Geometry check sheet. Reference: the model listing, model coordinates, mm. Face numbers are marked on the shaded views. A direction names the side the tool comes from. Round coordinates to 2 decimals unless told otherwise and drop trailing zeros. Write each loop counter-clockwise with the first axis right and the second up, starting at its lowest first coordinate (ties: lowest second). Pieces come first, ordered by that corner, then holes. Notation, with made-up numbers: (-5.75, 41) -> (47.25, 41) arc R24 ccw to (47.25, 66) -> close; hole circle Ø11 at (-28, 8). An arc over 180 degrees is marked (long way). One line per question, with ' | ' between items.
```python
from build123d import *

# Parameters (mm, degrees)
BOSS_EXTRUDE1_DEPTH       = 5
CUT_EXTRUDE1_DEPTH        = 0.5
CUT_EXTRUDE2_DEPTH        = 3
M3X0_5_TAPPED_HOLE1_D     = 2.5
M3X0_5_TAPPED_HOLE1_DEPTH = 7.5
M3X0_5_TAPPED_HOLE1_TIP   = 0.751075774
FILLET1_R                 = 0.5


with BuildPart() as part:
    # Sketch1 → Boss-Extrude1 (new body)
    with BuildSketch(Plane(origin=(0, 0, 0), x_dir=(1, 0, 0), z_dir=(0, 1, 0))):
        with BuildLine():
            Line((-30, 11), (-6, 11))
            Line((-6, 11), (-6, 0))
            ThreePointArc((-6, 0), (0, -6), (6, 0))
            Line((6, 0), (6, 11))
            Line((6, 11), (40, 11))
            Line((40, 11), (40, -14))
            Line((40, -14), (-30, -14))
            Line((-30, -14), (-30, -2.5))
            Line((-30, -2.5), (-22, -2.5))
            ThreePointArc((-22, -2.5), (-19.5, 0), (-22, 2.5))
            Line((-22, 2.5), (-30, 2.5))
            Line((-30, 2.5), (-30, 11))
        make_face()
        with BuildLine():
            Line((22, 2.5), (30, 2.5))
            ThreePointArc((30, 2.5), (32.5, 0), (30, -2.5))
            Line((30, -2.5), (22, -2.5))
            ThreePointArc((22, -2.5), (19.5, 0), (22, 2.5))
        make_face(mode=Mode.SUBTRACT)
    extrude(amount=BOSS_EXTRUDE1_DEPTH)

    # Sketch2 → Cut-Extrude1 (cut)
    with BuildSketch(Plane.XZ):
        with BuildLine():
            Line((-9, 0), (-9, -11))
            Line((-9, -11), (9, -11))
            Line((9, -11), (9, 0))
            ThreePointArc((9, 0), (0, 9), (-9, 0))
        make_face()
    extrude(amount=-CUT_EXTRUDE1_DEPTH, mode=Mode.SUBTRACT)

    # Sketch3 → Cut-Extrude2 (cut)
    with BuildSketch(Plane.XZ):
        with BuildLine():
            Line((-11, 8), (-11, -5))
            ThreePointArc((-11, -5), (-14, -8), (-17, -5))
            Line((-17, -5), (-17, 8))
            ThreePointArc((-17, 8), (-14, 11), (-11, 8))
        make_face()
        with BuildLine():
            Line((18, 8), (18, -5))
            ThreePointArc((18, -5), (14.5, -8.5), (11, -5))
            Line((11, -5), (11, 8))
            ThreePointArc((11, 8), (14.5, 11.5), (18, 8))
        make_face()
        with BuildLine():
            Line((38.85, 7.5), (38.85, -5))
            ThreePointArc((38.85, -5), (36.35, -7.5), (33.85, -5))
            Line((33.85, -5), (33.85, 7.5))
            ThreePointArc((33.85, 7.5), (36.35, 10), (38.85, 7.5))
        make_face()
    extrude(amount=-CUT_EXTRUDE2_DEPTH, mode=Mode.SUBTRACT)

    # M3x0.5 Tapped Hole1
    with Locations(Plane.XY.offset(14)):
        with Locations((30, 2.5)):
            Hole(M3X0_5_TAPPED_HOLE1_D / 2, depth=M3X0_5_TAPPED_HOLE1_DEPTH)
            with Locations((0, 0, -(M3X0_5_TAPPED_HOLE1_DEPTH + M3X0_5_TAPPED_HOLE1_TIP / 2))):  # 118° drill point
                Cone(0, M3X0_5_TAPPED_HOLE1_D / 2, M3X0_5_TAPPED_HOLE1_TIP, mode=Mode.SUBTRACT)

    # Fillet1
    fillet1_edges = [part.edges().sort_by_distance(p)[0] for p in [
        (40, 2.5, -11),
        (40, 2.5, 14),
        (-30, 2.5, 14),
        (-30, 2.5, -11),
        (-6, 2.75, -11),
        (6, 2.75, -11),
    ]]
    fillet(fillet1_edges, radius=FILLET1_R)


solid = part.part
```
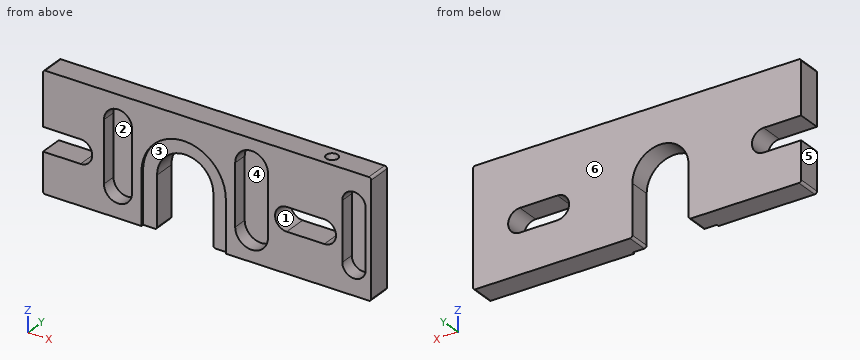
(1) Access from +Z, -Z, +X, -X, +Y, -Y to the whole of each face (thin tool, end or side, straight path). Record for the marked faces 1, 2 and 3.
Resolved:
face 1: +Y, -Y | face 2: -Y | face 3: -Z, -Y
(2) Sectioned sample at D-D on x = 0. Record the cut outline in (y, z).
Resolved:
outline: (0, 9) -> (0.5, 9) -> (0.5, 6) -> (5, 6) -> (5, 14) -> (0, 14) -> close
(3) Sectioned sample at B-B on x = 36.35. Record the cut outline in (y, z).
Resolved:
outline: (0, -11) -> (5, -11) -> (5, 14) -> (0, 14) -> (0, 10) -> (3, 10) -> (3, -7.5) -> (0, -7.5) -> close
(4) Sectioned sample at C-C on z = 3.5. Record the cut outline in (x, y), then the cut area to 3 significant figures.
Resolved:
outline: (-30, 0) -> (-17, 0) -> (-17, 3) -> (-11, 3) -> (-11, 0) -> (-8.29, 0) -> (-8.29, 0.5) -> (-4.87, 0.5) -> (-4.87, 5) -> (-30, 5) -> close; (4.87, 0.5) -> (8.29, 0.5) -> (8.29, 0) -> (11, 0) -> (11, 3) -> (18, 3) -> (18, 0) -> (33.85, 0) -> (33.85, 3) -> (38.85, 3) -> (38.85, 0) -> (40, 0) -> (40, 5) -> (4.87, 5) -> close | area: 244 mm2
(5) Sectioned sample at A-A on z = -9.25. Record the cut outline in (x, y), then the cut area to 3 significant figures.
Resolved:
outline: (-30, 0) -> (-9, 0) -> (-9, 0.5) -> (-6, 0.5) -> (-6, 5) -> (-30, 5) -> close; (6, 0.5) -> (9, 0.5) -> (9, 0) -> (40, 0) -> (40, 5) -> (6, 5) -> close | area: 287 mm2
(6) Go/stop test with flat-tipped pins: pin 1 (14.5 mm diameter, centred on x = 2, z = -4, fed in from -Y); pin 2 (1 mm diameter, centred on x = -4.5, y = 2.5, fed in from -Z); pin 3 (0.9 mm diameter, centred on y = 2, z = 0.5, fed in from -X); pin 4 (2 mm diameter, centred on x = 14.5, z = -0.5, fed in from -Y). Record where each tip stops, or that it passes through.
Resolved:
pin 1: stops at y = 0 | pin 2: stops at z = 3.32 | pin 3: stops at x = -19.69 | pin 4: stops at y = 3
(7) Draft check along X on the marked faces 4, 5 and 6. Enter one of: +X half, -X half, draft (parallel to the pull), parting line (faces both ways), or undercut.
Resolved:
face 4: undercut | face 5: -X half | face 6: draft
(8) Material ranges on line 1 (X direction, y = 0.75, z = -9.25); line 2 (Z direction, x = 14.5, y = 2.65); line 3 (X direction, y = 2.5, z = 9), recorded low to high.
Resolved:
line 1: x = -30 to -6, 6 to 40 | line 2: z = -11 to -8.5, 11.5 to 14 | line 3: x = -30 to -16.83, -11.17 to 11.15, 17.85 to 28.75, 31.25 to 34.35, 38.35 to 40
